from build123d import *

# Parameters (mm, degrees)
SCHIZZO1_R                             = 30
SCHIZZO1_R_2                           = 3
ESTRUSIONE_ESTRUSIONE1_DEPTH           = 2
FORO_SVASATO_PER_VITE_M2_1_D           = 2.4
FORO_SVASATO_PER_VITE_M2_1_DEPTH       = 6
FORO_SVASATO_PER_VITE_M2_1_CSINK_D     = 4.4
FORO_SVASATO_PER_VITE_M2_1_CSINK_ANGLE = 90
FORO_SVASATO_PER_VITE_M2_1_TIP         = 0.721032743


with BuildPart() as part:
    # Schizzo1 → Estrusione-Estrusione1 (new body)
    with BuildSketch(Plane.XY):
        Circle(SCHIZZO1_R)
        Circle(SCHIZZO1_R_2, mode=Mode.SUBTRACT)
    extrude(amount=ESTRUSIONE_ESTRUSIONE1_DEPTH)

    # Foro svasato per Vite M2-1
    with Locations(Plane(origin=(0, 0, 0), x_dir=(-1, 0, 0), z_dir=(0, 0, -1))):
        with Locations((0, -26), (-25, 3), (25, 3)):
            CounterSinkHole(FORO_SVASATO_PER_VITE_M2_1_D / 2, FORO_SVASATO_PER_VITE_M2_1_CSINK_D / 2, depth=FORO_SVASATO_PER_VITE_M2_1_DEPTH, counter_sink_angle=FORO_SVASATO_PER_VITE_M2_1_CSINK_ANGLE)
            with Locations((0, 0, -(FORO_SVASATO_PER_VITE_M2_1_DEPTH + FORO_SVASATO_PER_VITE_M2_1_TIP / 2))):  # 118° drill point
                Cone(0, FORO_SVASATO_PER_VITE_M2_1_D / 2, FORO_SVASATO_PER_VITE_M2_1_TIP, mode=Mode.SUBTRACT)


solid = part.part
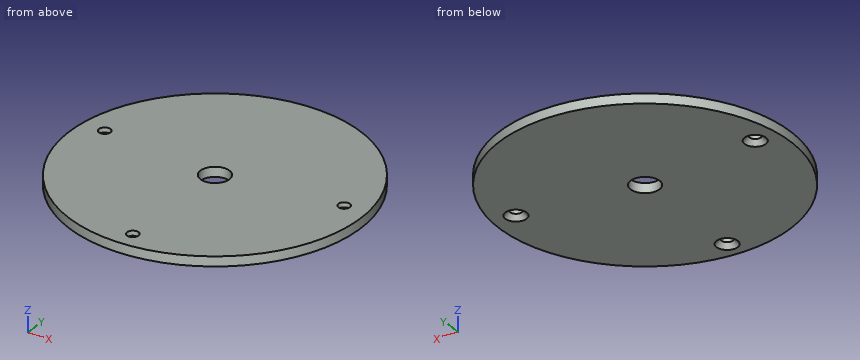
The listing builds one solid part. Answer for the finished solid, in the listing's coordinates (mm). Round coordinates to 2 decimals unless told otherwise and drop trailing zeros. Write each loop counter-clockwise with the first axis right and the second up, starting at its lowest first coordinate (ties: lowest second). Pieces come first, ordered by that corner, then holes. Notation, with made-up numbers: (26, 29.5) - (79, 29.5) arc R20 ccw to (79, 50.5) - close; hole circle Ø4 at (-16, -20.75). An arc over 180 degrees is marked (long way). Use one line per item in the form item = value. Start each with the question number.
Item 1: A cutting plane is placed at D-D (x = 25). Write down the section's boundary in (y, z), plus the area to 3 significant figures.
Item 2: Flat-ended cylindrical pins translate along their axes: pin 1 Ø3 at (x, y) = (25, 3) entering from +Z; pin 2 Ø3 at (x, y) = (0, -26) entering from -Z. Find the tip coordinate at first contact, or state that the pin passes through.
Item 3: A cutting plane is placed at B-B (y = 0). Write down the section's boundary in (x, z), plus the area to 3 significant figures.
Item 4: A cutting plane is placed at C-C (z = 0.3). Write down the section's boundary in (x, y), plus the area to 3 significant figures.
Item 5: Find the intervals of material crossed by line 1 (Y direction, x = 0, z = 1.7); line 2 (X direction, y = 3.5, z = 1.3); line 3 (X direction, y = -26, z = 1.25), in increasing order. Write a range as [from, to].
Item 6: A cutting plane is placed at A-A (x = 0). Write down the section's boundary in (y, z).
The answers:
q1.outline = (-16.58, 0) - (0.8, 0) - (1.8, 1) - (1.8, 2) - (-16.58, 2) - close; (4.2, 1) - (5.2, 0) - (16.58, 0) - (16.58, 2) - (4.2, 2) - close
q1.area = 60.5 mm^2
q2.pin_1 = 2
q2.pin_2 = 0.7
q3.outline = (-30, 0) - (-3, 0) - (-3, 2) - (-30, 2) - close; (3, 0) - (30, 0) - (30, 2) - (3, 2) - close
q3.area = 108 mm^2
q4.outline = circle Ø60 at (0, 0); hole circle Ø3.8 at (-25, 3); hole circle Ø6 at (0, 0); hole circle Ø3.8 at (0, -26); hole circle Ø3.8 at (25, 3)
q4.area = 2,770 mm^2
q5.line_1 = [-30, -27.2], [-24.8, -3], [3, 30]
q5.line_2 = [-29.8, -26.09], [-23.91, 23.91], [26.09, 29.8]
q5.line_3 = [-14.97, -1.2], [1.2, 14.97]
q6.outline = (-30, 0) - (-28.2, 0) - (-27.2, 1) - (-27.2, 2) - (-30, 2) - close; (-24.8, 1) - (-23.8, 0) - (-3, 0) - (-3, 2) - (-24.8, 2) - close; (3, 0) - (30, 0) - (30, 2) - (3, 2) - close
